from build123d import *

# Parameters (mm, degrees)
SKETCH1_R           = 7
BOSS_EXTRUDE1_DEPTH = 1
SKETCH2_R           = 7
BOSS_EXTRUDE2_DEPTH = 1.5
BOSS_EXTRUDE2_TAPER = 45
SKETCH3_R           = 5
CUT_EXTRUDE1_DEPTH  = 1
CUT_EXTRUDE1_DRAFT  = -45
SKETCH4_R           = 6
BOSS_EXTRUDE3_DEPTH = 23
NUT_DEPTH           = 2


with BuildPart() as part:
    # Sketch1 → Boss-Extrude1 (new body)
    with BuildSketch(Plane.XY):
        Circle(SKETCH1_R)
    extrude(amount=BOSS_EXTRUDE1_DEPTH)

    # Sketch2 → Boss-Extrude2 (add)
    with BuildSketch(Plane.XY.offset(1)):
        Circle(SKETCH2_R)
    extrude(amount=BOSS_EXTRUDE2_DEPTH, taper=BOSS_EXTRUDE2_TAPER)


with BuildPart() as cut_extrude1_tool:
    # Sketch3 → Cut-Extrude1 (with draft: the straight prism first)
    with BuildSketch(Plane.XY.offset(2.5)):
        Circle(SKETCH3_R)
    extrude(amount=-CUT_EXTRUDE1_DEPTH)
    # Cut-Extrude1: the draft: its side faces are tilted about the plane it starts from
    cut_extrude1_sides = [cut_extrude1_tool.faces().sort_by_distance(p)[0] for p in [
        (-5, 0, 2),
    ]]
    draft(cut_extrude1_sides, Plane.XY.offset(2.5), CUT_EXTRUDE1_DRAFT)


with BuildPart() as part_1:
    add(part.part)

    # Cut-Extrude1: cut by cut_extrude1_tool
    add(cut_extrude1_tool.part, mode=Mode.SUBTRACT)

    # Sketch4 → Boss-Extrude3 (add)
    with BuildSketch(Plane.XY):
        Circle(SKETCH4_R)
    extrude(amount=-BOSS_EXTRUDE3_DEPTH)

    # Sketch5 → Nut (add)
    with BuildSketch(Plane.XY.offset(-2)):
        Polygon((0, 8.025168742), (-6.95, 4.012584371), (-6.95, -4.012584371), (0, -8.025168742), (6.95, -4.012584371), (6.95, 4.012584371), align=None)
    extrude(amount=-NUT_DEPTH)


solid = part_1.part
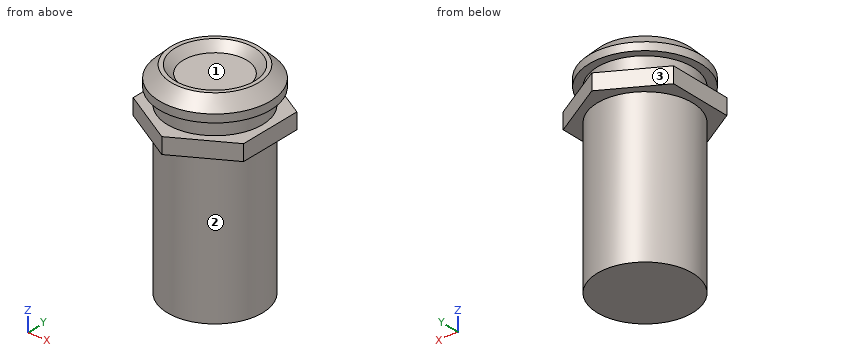
Can you work these out from the model? Positions are in its coordinate system, mm. Face numbers are marked on the shaded views. Coordinates: 2 decimals unless noted, no trailing zeros. Write each loop counter-clockwise with the first axis right and the second up, starting at its lowest first coordinate (ties: lowest second). Pieces come first, ordered by that corner, then holes. Notation, with made-up numbers: M 69,43 L 98,43 A19 ccw 98,79 Z; hole C 49.25,25.5 d5. An arc over 180 degrees is marked long. Use one line per item in the form item = value.
Q1. I need wall thicknesses on line 1 along Z through (x, y) = (1.5, -2.25); line 2 along Z through (x, y) = (5.25, 3); line 3 along Y through (x, z) = (0.25, 1.75) (3 decimals). Which ranges of each line are inside material? Lowest first, please. Write a range as from..to.
Model answer:
line_1 = -23..1.5
line_2 = -4..-2, 0..1.95
line_3 = -6.245..-4.243, 4.243..6.245
Q2. If we section it at B-B (z = -15.5): Write out the boundary of the cut face in (x, y), then the cut area to 3 significant figures.
Model answer:
outline = C 0,0 d12
area = 113 mm^2
Q3. If we section it at A-A (y = 0): Write out the boundary of the cut face in (x, z).
Model answer:
outline = M -7,0 L -6,0 L -6,-2 L -6.95,-2 L -6.95,-4 L -6,-4 L -6,-23 L 6,-23 L 6,-4 L 6.95,-4 L 6.95,-2 L 6,-2 L 6,0 L 7,0 L 7,1 L 5.5,2.5 L 5,2.5 L 4,1.5 L -4,1.5 L -5,2.5 L -5.5,2.5 L -7,1 Z
Q4. For P1, Ø4, axis at y = -2.5, z = -10.5, coming from the +X side; P2, Ø2, axis at x = 4, z = -16, coming from the +Y side; P3, Ø3, axis at y = 2.5, z = -17.5, coming from the -X side, each with a flat end and sliding along its axis, tell me the tip position at first contact or that it passes through.
Model answer:
P1 = 5.98
P2 = 5.2
P3 = -5.92
Q5. We'd pull the mould along X, two halves only. Please class the marked faces 1, 2 and 3: +X half, -X half, draft (parallel to the pull), parting line (faces both ways), or undercut.
Model answer:
face_1 = undercut
face_2 = parting line
face_3 = -X half
